Here's how the part is built. I have some questions about the finished solid (model axes, mm). Face numbers are marked on the shaded views. A direction names the side the tool comes from. Round coordinates to 2 decimals unless told otherwise and drop trailing zeros. Order: outer loops, then holes, each group sorted by start corner. A loop starts at its lowest first (then second) coordinate and runs counter-clockwise, first axis right, second up. Notation, with made-up numbers: (-8, 58) -> (6, 58) arc R19 ccw to (6, 63) -> close; hole circle Ø2 at (15.25, 14). An arc over 180 degrees is marked (long way). Use a Markdown table: item, result. Add a question column.
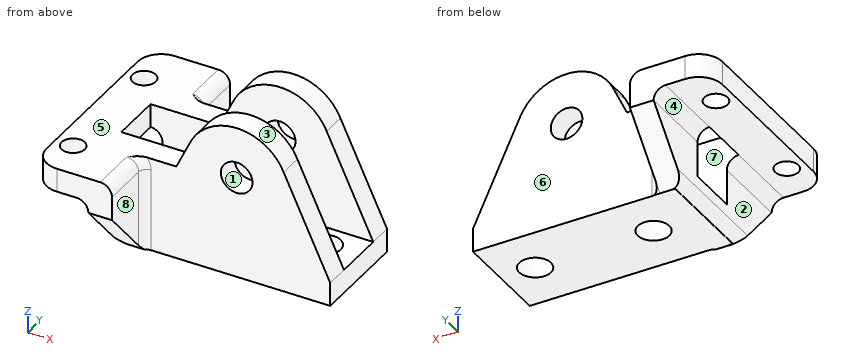
from build123d import *

# Parameters (mm, degrees)
ESQUISSE1_W             = 23.695260015
ESQUISSE1_H             = 12.6
ESQUISSE1_R             = 2
BOSS_EXTRU_1_DEPTH      = 3
ESQUISSE3_R             = 2
BOSS_EXTRU_2_DEPTH      = 12.6
BOSS_EXTRU_4_DEPTH      = 6.7
BOSS_EXTRU_4_DEPTH_BACK = 19.5
ENL_V_MAT_EXTRU_2_DEPTH = 3
ESQUISSE8_W             = 8.43757856
ESQUISSE8_H             = 12
BOSS_EXTRU_5_DEPTH      = 12.6
ESQUISSE5_W             = 20.633758591
ESQUISSE5_H             = 6.5
ENL_V_MAT_EXTRU_1_DEPTH = 28.2
CONG_3_R                = 1
ESQUISSE9_R             = 2
ENL_V_MAT_EXTRU_3_DEPTH = 3.6
ESQUISSE11_R            = 1.47
ENL_V_MAT_EXTRU_4_DEPTH = 3.6
CONG_4_R                = 3


with BuildPart() as part:
    # Esquisse1 → Boss.-Extru.1 (new body)
    with BuildSketch(Plane.XY):
        with Locations((-5.99209908, 12.295954438)):
            Rectangle(ESQUISSE1_W, ESQUISSE1_H)
        with Locations((-13.489729087, 12.425985115)):
            Circle(ESQUISSE1_R, mode=Mode.SUBTRACT)
        with Locations((1.510270913, 12.425985115)):
            Circle(ESQUISSE1_R, mode=Mode.SUBTRACT)
    extrude(amount=BOSS_EXTRU_1_DEPTH)

    # Esquisse3 → Boss.-Extru.2 (add)
    with BuildSketch(Plane.XZ.offset(-5.995954438)):
        with BuildLine():
            Line((-17.839729087, 3), (5.855530928, 3))
            Line((5.855530928, 3), (-0.041538546, 15.615497913))
            ThreePointArc((-0.041538546, 15.615497913), (-5.99209908, 19.5), (-11.942659613, 15.615497913))
            Line((-11.942659613, 15.615497913), (-17.839729087, 3))
        make_face()
        with Locations(Location((-5.99209908, 13, 0), (0, 0, 270))):
            Circle(ESQUISSE3_R, mode=Mode.SUBTRACT)
    extrude(amount=-BOSS_EXTRU_2_DEPTH)

    # Esquisse6 → Boss.-Extru.4 (add, two sides: drawn at the far end of the back side and taken through both)
    with BuildSketch(Plane(origin=(0, 18.595954438, 0), x_dir=(1, 0, 0), z_dir=(0, 1, 0)).offset(-BOSS_EXTRU_4_DEPTH_BACK)):
        with BuildLine():
            Line((-17.839729087, -3), (-17.839729087, 0))
            Line((-17.839729087, 0), (-19.339729087, 0))
            ThreePointArc((-19.339729087, 0), (-20.400389259, -0.439339828), (-20.839729087, -1.5))
            Line((-20.839729087, -1.5), (-20.839729087, -7.5))
            ThreePointArc((-20.839729087, -7.5), (-21.279068915, -8.560660172), (-22.339729087, -9))
            Line((-22.339729087, -9), (-27.839729087, -9))
            Line((-27.839729087, -9), (-27.839729087, -12))
            Line((-27.839729087, -12), (-19.944823835, -12))
            Line((-19.944823835, -12), (-19.339729087, -12))
            ThreePointArc((-19.339729087, -12), (-18.279068915, -11.560660172), (-17.839729087, -10.5))
            Line((-17.839729087, -10.5), (-17.839729087, -8.3919439))
            Line((-17.839729087, -8.3919439), (-17.839729087, -3))
        make_face()
    extrude(amount=BOSS_EXTRU_4_DEPTH + BOSS_EXTRU_4_DEPTH_BACK)

    # Esquisse7 → Enlèv. mat.-Extru.2 (cut)
    with BuildSketch(Plane.ZY.offset(20.839729087)):
        Polygon((-6.140344815, 12.195954438), (-6.42704232, 7.753847566), (-3.772480019, -6.539015172), (6.059758422, -5.019044791), (7.5, -0.904045562), (-0.069254369, 5.816985209), (-0.466179864, 12.195954438), (-0.069254369, 18.574923667), (7.5, 25.295954438), (6.059758422, 29.410953667), (-3.772480019, 30.930924048), (-6.42704232, 16.638061311), align=None)
    extrude(amount=-ENL_V_MAT_EXTRU_2_DEPTH, mode=Mode.SUBTRACT)

    # Esquisse8 → Boss.-Extru.5 (add)
    with BuildSketch(Plane(origin=(0, 5.995954438, 0), x_dir=(-1, 0, 0), z_dir=(0, -1, 0))):
        with Locations((15.523391269, -6)):
            Rectangle(ESQUISSE8_W, ESQUISSE8_H)
    extrude(amount=-BOSS_EXTRU_5_DEPTH)

    # Esquisse5 → Enlèv. mat.-Extru.1 (cut)
    with BuildSketch(Plane(origin=(5.855530928, 0, 0), x_dir=(0, 0, -1), z_dir=(1, 0, 0))):
        with Locations((-13.316879296, 12.295954438)):
            Rectangle(ESQUISSE5_W, ESQUISSE5_H)
    extrude(amount=-ENL_V_MAT_EXTRU_1_DEPTH, mode=Mode.SUBTRACT)

    # Congé3
    # the kernel refuses this fillet: 1 mm, written as the material it adds along each edge
    with BuildSketch(Plane(origin=(-19.339729087, 18.595954438, 10.5), x_dir=(1, 0, 0), z_dir=(0, 0, -1))) as cong_3_piece_1_section:
        with BuildLine():
            CenterArc((1.5 + CONG_3_R, -CONG_3_R), CONG_3_R, 90, 90)
            Line((1.5, -CONG_3_R), (1.5, 0))
            Line((1.5, 0), (1.5 + CONG_3_R, 0))
        make_face()
    cong_3_piece_1 = revolve(axis=Axis((-19.339729087, 18.595954438, 10.5), (0, -1, 0)), revolution_arc=185.531326158, mode=Mode.PRIVATE)
    cong_3_piece_1 = split(cong_3_piece_1, bisect_by=Plane(origin=(-17.625243019, 18.758648555, 12), z_dir=(0, 0, -1)), keep=Keep.TOP, mode=Mode.PRIVATE)
    add(cong_3_piece_1)
    with BuildSketch(Plane(origin=(-19.339729087, 5.995954438, 10.5), x_dir=(1, 0, 0), z_dir=(0, 0, -1))) as cong_3_piece_2_section:
        with BuildLine():
            CenterArc((1.5 + CONG_3_R, CONG_3_R), CONG_3_R, 180, 90)
            Line((1.5 + CONG_3_R, 0), (1.5, 0))
            Line((1.5, 0), (1.5, CONG_3_R))
        make_face()
    cong_3_piece_2 = revolve(axis=Axis((-19.339729087, 5.995954438, 10.5), (0, -1, 0)), revolution_arc=185.531326158, mode=Mode.PRIVATE)
    cong_3_piece_2 = split(cong_3_piece_2, bisect_by=Plane(origin=(-18.22928563, 5.709154501, 12), z_dir=(0, 0, -1)), keep=Keep.TOP, mode=Mode.PRIVATE)
    add(cong_3_piece_2)
    with BuildSketch(Plane(origin=(-17.839729087, 18.595954438, 0), x_dir=(1, 0, 0), z_dir=(0, 0, 1))) as cong_3_piece_3_section:
        with BuildLine():
            CenterArc((CONG_3_R, CONG_3_R), CONG_3_R, 180, 90)
            Line((0, CONG_3_R), (0, 0))
            Line((0, 0), (CONG_3_R, 0))
        make_face()
    cong_3_piece_3 = extrude(amount=10.5, mode=Mode.PRIVATE)
    cong_3_piece_3 = split(cong_3_piece_3, bisect_by=Plane(origin=(-17.614169597, 21.372960388, 3.081906873), z_dir=(0, -0.7477621735263639, 0.6639666647077458)), keep=Keep.TOP, mode=Mode.PRIVATE)
    add(cong_3_piece_3)
    with BuildSketch(Plane(origin=(-17.839729087, 5.995954438, 0), x_dir=(1, 0, 0), z_dir=(0, 0, 1))) as cong_3_piece_4_section:
        with BuildLine():
            CenterArc((CONG_3_R, -CONG_3_R), CONG_3_R, 90, 90)
            Line((0, -CONG_3_R), (0, 0))
            Line((0, 0), (CONG_3_R, 0))
        make_face()
    cong_3_piece_4 = extrude(amount=10.5, mode=Mode.PRIVATE)
    cong_3_piece_4 = split(cong_3_piece_4, bisect_by=Plane(origin=(-17.615177954, 3.13865295, 2.947095183), z_dir=(0, 0.747762173526364, 0.6639666647077457)), keep=Keep.TOP, mode=Mode.PRIVATE)
    add(cong_3_piece_4)

    # Esquisse9 → Enlèv. mat.-Extru.3 (cut)
    with BuildSketch(Plane(origin=(0, 0, 0), x_dir=(-1, 0, 0), z_dir=(0, 0, -1))):
        with Locations((13.489729087, 12.425985115)):
            Circle(ESQUISSE9_R)
    extrude(amount=-ENL_V_MAT_EXTRU_3_DEPTH, mode=Mode.SUBTRACT)

    # Esquisse11 → Enlèv. mat.-Extru.4 (cut)
    with BuildSketch(Plane(origin=(0, 0, 9), x_dir=(-1, 0, 0), z_dir=(0, 0, -1))):
        with Locations((25.570191421, 4.024422561)):
            Circle(ESQUISSE11_R)
        with Locations((25.570191421, 19.752422561)):
            Circle(ESQUISSE11_R)
    extrude(amount=-ENL_V_MAT_EXTRU_4_DEPTH, mode=Mode.SUBTRACT)

    # Congé4
    cong_4_edges = [part.edges().sort_by_distance(p)[0] for p in [
        (-27.839729087, 25.295954438, 10.5),
        (-27.839729087, -0.904045562, 10.5),
    ]]
    fillet(cong_4_edges, radius=CONG_4_R)


solid = part.part
(1) I want a section at A-A on z = 14.25. List the corners of the cut face in (x, y) for me, and give its area (3 significant figures).
(2) On a 3-axis mill with a long thin cutter (end or side, diameter ignored), from which of +Z, -Z, +X, -X, +Y, -Y can I reach the whole of each face in a straight line? I mean the marked faces 5, 6, 7 and 8. Say none if no direction works.
(3) I want a section at D-D on x = -4.5. List the corners of the cut face in (y, z) for me.
(4) Please list where these lines run through material, in increasing order: probe 1 along Y at (x, z) = (-18.5, 11.5); probe 2 along Y at (x, z) = (-3, 5); probe 3 along X at (y, z) = (12, 11.5). Write a range as from..to.
(5) I want a section at B-B on x = 3. List the corners of the cut face in (y, z) for me.
(6) I'm going to push flat-ended pins straight in: P1, Ø6.5, axis at y = 6.5, z = 4, coming from the -X side; P2, Ø2, axis at x = -0.5, z = 15.5, coming from the -Y side; P3, Ø6, axis at x = -14.5, z = 8, coming from the -Y side. Where does each tip first touch, or does it pass through?
(7) If we mould it in two halves opening along Z, with no side actions, what happens to the marked faces 1, 2, 3 and 4? For each: pulls with the +Z half, pulls with the -Z half, needs draft (parallel to the pull), parting line crosses it, or undercut.
(8) I want a section at C-C on y = 13.75. List the corners of the cut face in (x, z) for me (3 decimals).
Output:
| question | item | result |
|---|---|---|
| 1 | outline | (-12.58, 6) -> (-7.55, 6) -> (-7.55, 9.05) -> (-12.58, 9.05) -> close; (-12.58, 15.55) -> (-7.55, 15.55) -> (-7.55, 18.6) -> (-12.58, 18.6) -> close; (-4.43, 6) -> (0.6, 6) -> (0.6, 9.05) -> (-4.43, 9.05) -> close; (-4.43, 15.55) -> (0.6, 15.55) -> (0.6, 18.6) -> (-4.43, 18.6) -> close |
| 1 | area | 61.3 mm² |
| 2 | face 5 | +Z, -X, +Y, -Y |
| 2 | face 6 | +Z, -Z, +X, +Y |
| 2 | face 7 | +Z, +X |
| 2 | face 8 | +Z, -Z, +X, -Y |
| 3 | outline | (6, 0) -> (18.6, 0) -> (18.6, 11.67) -> (15.55, 11.67) -> (15.55, 3) -> (9.05, 3) -> (9.05, 11.67) -> (6, 11.67) -> close; (6, 14.33) -> (9.05, 14.33) -> (9.05, 19.33) -> (6, 19.33) -> close; (15.55, 14.33) -> (18.6, 14.33) -> (18.6, 19.33) -> (15.55, 19.33) -> close |
| 4 | probe 1 | -0.9..9.05, 15.55..25.3 |
| 4 | probe 2 | 6..9.05, 15.55..18.6 |
| 4 | probe 3 | -27.84..-22.34 |
| 5 | outline | (6, 0) -> (11.09, 0) -> (11.09, 3) -> (9.05, 3) -> (9.05, 9.11) -> (6, 9.11) -> close; (13.76, 0) -> (18.6, 0) -> (18.6, 9.11) -> (15.55, 9.11) -> (15.55, 3) -> (13.76, 3) -> close |
| 6 | P1 | x = -20.84 |
| 6 | P2 | y = 6 |
| 6 | P3 | y = 5.75 |
| 7 | face 1 | undercut |
| 7 | face 2 | needs draft |
| 7 | face 3 | pulls with the +Z half |
| 7 | face 4 | pulls with the -Z half |
| 8 | outline | (-27.84, 9) -> (-22.344, 9) -> (-22.344, 12) -> (-27.84, 12) -> close; (-20.84, 1.5) arc R1.5 ccw to (-19.742, 0.055) -> (-19.742, 0) -> (-14.989, 0) -> (-14.989, 3) -> (-20.84, 3) -> close; (-11.991, 0) -> (0.011, 0) -> (0.011, 3) -> (-11.991, 3) -> close; (3.009, 0) -> (5.856, 0) -> (5.856, 3) -> (3.009, 3) -> close |
